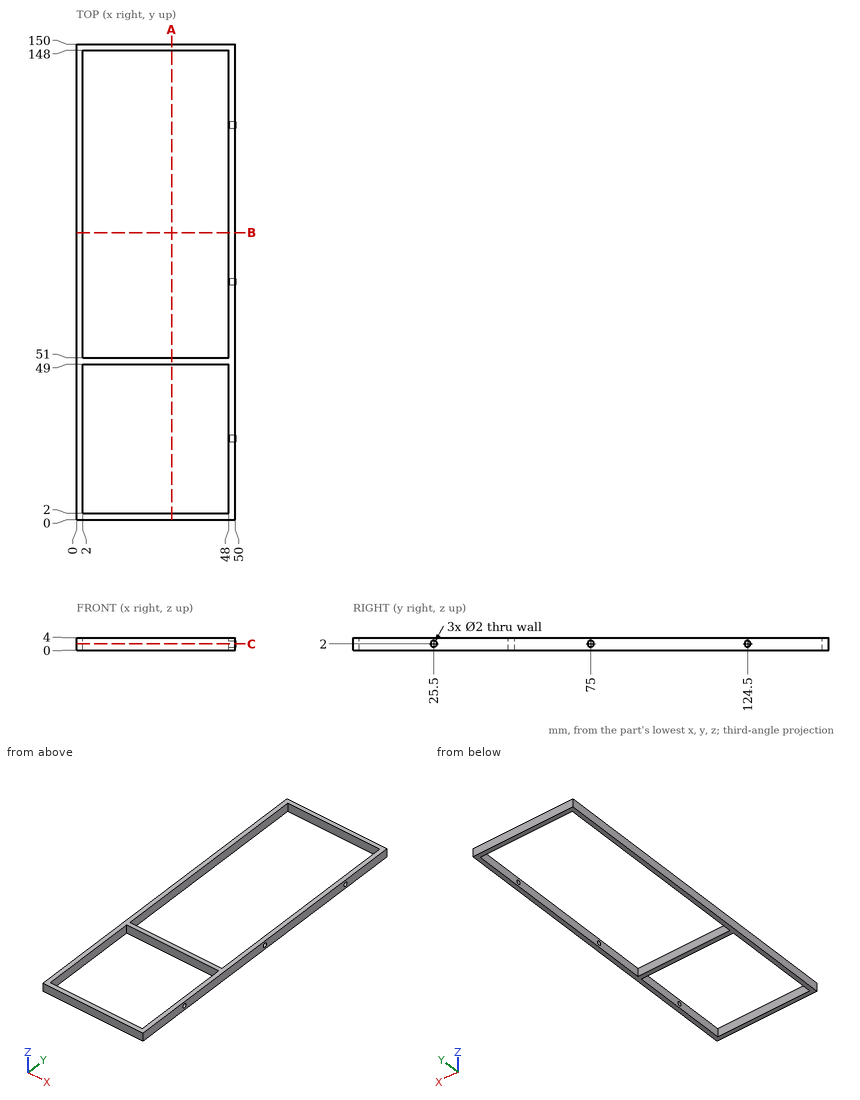
Geometry check sheet. Reference: drawing and pictorial views, mm from the part's lowest x, y, z. Give positions to 0.01 mm unless a question says otherwise; leave off trailing zeros. Order: outer loops, then holes, each group sorted by start corner. A loop starts at its lowest first (then second) coordinate and runs counter-clockwise, first axis right, second up. Notation, with made-up numbers: M 41.5,-39 L 59.5,-39 A15 ccw 59.5,-28 Z; hole C -17.5,70.25 d4. An arc over 180 degrees is marked long. Return JSON: item names as keys, results as strings. Group by question number.
1) Section check A-A on x = 30. Record the cut outline in (y, z), and give its area (3 significant figures).
2) Section check B-B on y = 90.5. Record the cut outline in (x, z), and give its area (3 significant figures).
3) Scan lines: line 1 (Y direction, x = 8.5, z = 1.6); line 2 (X direction, y = 90, z = 2.9); line 3 (Z direction, x = 49, y = 75). Record each from-to range of solid material in increasing order.
4) Section check C-C on z = 2. Record the cut outline in (x, y), and give its area (3 significant figures).
5) Go/stop test with a flat-tipped pin: pin 1 Ø1.8 at (y, z) = (75, 2) entering from +X. Record where the tip stops, or that it passes through.
Answer block:
{
 "1": {"outline": "M 0,0 L 2,0 L 2,4 L 0,4 Z; M 49,0 L 51,0 L 51,4 L 49,4 Z; M 148,0 L 150,0 L 150,4 L 148,4 Z", "area": "24.0 mm^2"},
 "2": {"outline": "M 0,0 L 2,0 L 2,4 L 0,4 Z; M 48,0 L 50,0 L 50,4 L 48,4 Z", "area": "16.0 mm^2"},
 "3": {"line 1": "y = 0 to 2, 49 to 51, 148 to 150", "line 2": "x = 0 to 2, 48 to 50", "line 3": "z = 0 to 1, 3 to 4"},
 "4": {"outline": "M 0,0 L 50,0 L 50,24.5 L 48,24.5 L 48,2 L 2,2 L 2,49 L 48,49 L 48,26.5 L 50,26.5 L 50,74 L 48,74 L 48,51 L 2,51 L 2,148 L 48,148 L 48,125.5 L 50,125.5 L 50,150 L 0,150 Z; M 48,76 L 50,76 L 50,123.5 L 48,123.5 Z", "area": "864 mm^2"},
 "5": {"pin 1": "stops at x = 2"}
}
